```python
from build123d import *

# Parameters (mm, degrees)
SKETCH_1_W           = 7.62
SKETCH_1_H           = 7.62
EXTRUDE_1_DEPTH      = 10
CUT_EXTRUDE_1_DEPTH  = 8.5
EXTRUDE_2_DEPTH      = 4
EXTRUDE_2_DEPTH_BACK = 9
SKETCH_3_W           = 1
SKETCH_3_H           = 1


with BuildPart() as part:
    # 草图1 → 拉伸1 (new body)
    with BuildSketch(Plane(origin=(0, 0, 0), x_dir=(1, 0, 0), z_dir=(0, 1, 0))):
        Rectangle(SKETCH_1_W, SKETCH_1_H)
    extrude(amount=EXTRUDE_1_DEPTH)

    # 草图2 → 切除-拉伸1 (cut)
    with BuildSketch(Plane(origin=(0, 10, 0), x_dir=(-1, 0, 0), z_dir=(0, 1, 0))):
        with BuildLine():
            Line((-2.81, -3.81), (-2.81, -3.049818304))
            ThreePointArc((-2.81, -3.049818304), (-3.31, -1.905), (-2.81, -0.760181696))
            Line((-2.81, -0.760181696), (-2.81, 0.760181696))
            ThreePointArc((-2.81, 0.760181696), (-3.31, 1.905), (-2.81, 3.049818304))
            Line((-2.81, 3.049818304), (-2.81, 3.81))
            Line((-2.81, 3.81), (3.06, 3.81))
            Line((3.06, 3.81), (3.06, -3.81))
            Line((3.06, -3.81), (-2.81, -3.81))
        make_face()
    extrude(amount=-CUT_EXTRUDE_1_DEPTH, mode=Mode.SUBTRACT)

    # 草图3 → 拉伸2 (add, two sides: drawn at the far end of the back side and taken through both)
    with BuildSketch(Plane.XZ.offset(-EXTRUDE_2_DEPTH_BACK)):
        with Locations((-0.31, 1.905)):
            Rectangle(SKETCH_3_W, SKETCH_3_H)
        with Locations((-0.31, -1.905)):
            Rectangle(SKETCH_3_W, SKETCH_3_H)
    extrude(amount=EXTRUDE_2_DEPTH + EXTRUDE_2_DEPTH_BACK)


solid = part.part
```
Part model, mm, in its own coordinate system. A direction names the side the tool comes from. Round coordinates to 2 decimals unless told otherwise and drop trailing zeros. Write each loop counter-clockwise with the first axis right and the second up, starting at its lowest first coordinate (ties: lowest second). Pieces come first, ordered by that corner, then holes. Notation, with made-up numbers: (38, 68.5) -> (49, 68.5) arc R8 cw to (49, 82.5) -> close; hole circle Ø7 at (-13, 56.25). An arc over 180 degrees is marked (long way). Return JSON: item names as keys, results as strings. Group by question number.
Q1. Which spindle directions (+Z, -Z, +X, -X, +Y, -Y) get a long thin tool onto all of the face, cutting with end or side? Do faces 5 (the flat face through (0, 9, 2)), 6 (the flat face through (0, -2, 1.405)), 7 (the flat face through (0, -2, -2.405)), 8 (the flat face through (0, -2, 2.405)). Say none if no direction does.
Q2. Saw through at C-C on y = -2.5. Write the cut outline in (x, z) (3 decimals), plus the area to 3 significant figures.
Q3. Saw through at A-A on y = 2.25. Write the cut outline in (x, z) (3 decimals).
Q4. Mould opens along X. For faces 1 (the flat face through (0, 1, -3.81)), 2 (the flat face through (-0.81, -2, -2)), 3 (the flat face through (0, 5, -2.405)), 4 (the flat face through (0.19, -2, 2)) say: pulls with the +X half, pulls with the -X half, needs draft (parallel to the pull), parting line crosses it, or undercut.
Q5. Saw through at D-D on x = 2. Write the cut outline in (y, z).
Q6. Pin check, flat tips, straight feed: pin 1 (2 mm diameter, centred on x = 1.5, z = 1, fed in from +Y); pin 2 (2 mm diameter, centred on x = 0, z = -1.5, fed in from +Y); pin 3 (1.1 mm diameter, centred on y = -1.5, z = -2, fed in from -X). Stop position of each tip, or through.
Q7. Saw through at B-B on z = -0.25. Write the cut outline in (x, y), plus the area to 3 significant figures.
Q8. Probe L1, parallel to X at y = 4.25, z = -2; L2, parallel to Z at x = -0.75, y = 7 (3 decimals); L3, parallel to X at y = 6.5, z = -3.5. List the from-to ranges inside material, lowest first. Write a range as [from, to].
Answer:
{
 "1": {"face 5": "+Z, -Z, +Y", "face 6": "+X, -X, -Y", "face 7": "-Z, +X, -X, -Y", "face 8": "+Z, +X, -X, -Y"},
 "2": {"outline": "(-0.81, -2.405) -> (0.19, -2.405) -> (0.19, -1.405) -> (-0.81, -1.405) -> close; (-0.81, 1.405) -> (0.19, 1.405) -> (0.19, 2.405) -> (-0.81, 2.405) -> close", "area": "2.00 mm2"},
 "3": {"outline": "(-3.81, -3.81) -> (-3.06, -3.81) -> (-3.06, 3.81) -> (-3.81, 3.81) -> close; (-0.81, -2.405) -> (0.19, -2.405) -> (0.19, -1.405) -> (-0.81, -1.405) -> close; (-0.81, 1.405) -> (0.19, 1.405) -> (0.19, 2.405) -> (-0.81, 2.405) -> close; (2.81, -3.81) -> (3.81, -3.81) -> (3.81, 3.81) -> (2.81, 3.81) -> (2.81, 3.05) arc R1.561 cw to (2.81, 0.76) -> (2.81, -0.76) arc R1.561 cw to (2.81, -3.05) -> close"},
 "4": {"face 1": "needs draft", "face 2": "pulls with the -X half", "face 3": "undercut", "face 4": "pulls with the +X half"},
 "5": {"outline": "(0, -3.81) -> (1.5, -3.81) -> (1.5, 3.81) -> (0, 3.81) -> close"},
 "6": {"pin 1": "y = 1.5", "pin 2": "y = 9", "pin 3": "x = -0.81"},
 "7": {"outline": "(-3.81, 0) -> (3.81, 0) -> (3.81, 10) -> (2.81, 10) -> (2.81, 1.5) -> (-3.06, 1.5) -> (-3.06, 10) -> (-3.81, 10) -> close", "area": "26.3 mm2"},
 "8": {"L1": "[-3.81, -3.06], [-0.81, 0.19], [3.31, 3.81]", "L2": "[-2.405, -1.405], [1.405, 2.405]", "L3": "[-3.81, -3.06], [2.81, 3.81]"}
}
